from build123d import *

# Parameters (mm, degrees)
F2_R     = 3
F3_R     = 3
F4_R     = 7.243967
F5_DEPTH = 105.41


with BuildPart() as f1:
    # F0 (on Front) → F1 (revolve)
    with BuildSketch(Plane.XZ):
        Polygon((-12.904838, 16.591936), (-12.904838, 31.709034), (-12.904838, 46.826132), (-25.809675, 46.826132), (-25.809675, 56.412581), (-41.295484, 56.412581), (-41.295484, 63.418068), (-48.669677, 63.418068), (-48.669677, 49.038392), (-43.692097, 49.038392), (-43.692097, 31.709034), (-43.692097, 14.379676), (-48.669677, 14.379676), (-48.669677, 0), (-41.295484, 0), (-41.295484, 7.005487), (-25.809675, 7.005487), (-25.809675, 16.591936), align=None)
    revolve(axis=Axis((0, 0, 52.264599), (0, 0, 1)))

    # F2
    f2_edges = [f1.edges().sort_by_distance(p)[0] for p in [
        (43.692097, 0, 49.038392),
    ]]
    fillet(f2_edges, radius=F2_R)

    # F3
    f3_edges = [f1.edges().sort_by_distance(p)[0] for p in [
        (43.692097, 0, 14.379676),
    ]]
    fillet(f3_edges, radius=F3_R)

    # F4 (on Top) → F5 (cut)
    with BuildSketch(Plane.XY):
        with Locations((0, -33.43946)):
            Circle(F4_R)
        with Locations((-31.89178, -10.055439)):
            Circle(F4_R)
        with Locations((-19.180086, 27.392002)):
            Circle(F4_R)
        with Locations((20.356653, 26.529307)):
            Circle(F4_R)
        with Locations((31.422813, -11.436969)):
            Circle(F4_R)
    extrude(amount=F5_DEPTH, mode=Mode.SUBTRACT)


solid = f1.part
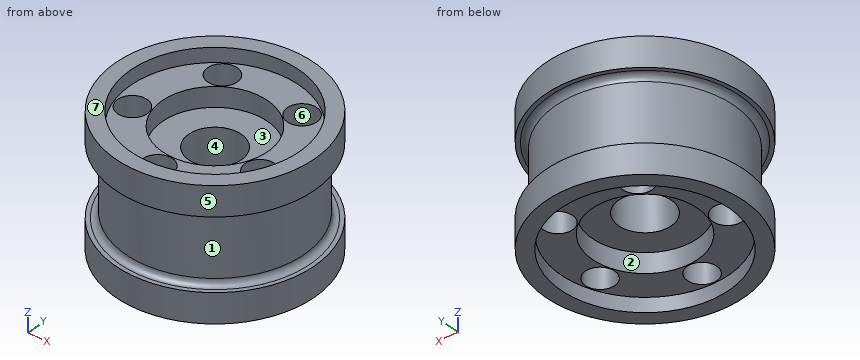
Could you check a few things on this model? Use its own coordinates, in mm. Face numbers are marked on the shaded views. A direction names the side the tool comes from. Give positions to 0.01 mm unless a question says otherwise; leave off trailing zeros. Order: outer loops, then holes, each group sorted by start corner. A loop starts at its lowest first (then second) coordinate and runs counter-clockwise, first axis right, second up.
1. I need wall thicknesses on L1, parallel to Y at x = 0, z = 52; L2, parallel to Y at x = 0, z = 59; L3, parallel to Y at x = 0, z = 23. Which ranges of each line are inside material? Lowest first, please.
2. Suppose I cut it at A-A (x = 0). Give the number of separate pieces and of enclosed holes in the cut face, plus the area to 3 significant figures.
3. We'd pull the mould along Y, two halves only. Please class the marked faces 5, 6 and 7: pulls with the +Y half, pulls with the -Y half, needs draft (parallel to the pull), parting line crosses it, or undercut.
4. For the marked faces 1, 2, 3 and 4, which set-ups out of +Z, -Z, +X, -X, +Y, -Y let a thin tool reach every point of the face, with its end or its side?
5. Will these pins go through, and if not, where does the flat tip stop? P1, Ø10, axis at y = 14.5, z = 28.5, coming from the -X side; P2, Ø13, axis at x = -31.89, y = -10.06, coming from the -Z side; P3, Ø1, axis at x = -16, z = 7.5, coming from the -Y side; P4, Ø10, axis at y = -31.5, z = 30.5, coming from the +X side.
6. Suppose I cut it at C-C (z = 32). List the corners of the cut face in (x, y) for me, plus the area to 3 significant figures.
7. Suppose I cut it at B-B (z = 4). List the corners of the cut face in (x, y) for me.
Solved:
1. L1: y = -48.67 to -40.68, -26.2 to -25.81, 25.81 to 48.67
1. L2: y = -48.67 to -41.3, 41.3 to 48.67
1. L3: y = -43.69 to -40.68, -26.2 to -12.9, 12.9 to 43.69
2. separate pieces: 3
2. enclosed holes: 0
2. area: 2,190 mm2
3. face 5: parting line crosses it
3. face 6: undercut
3. face 7: needs draft
4. face 1: none
4. face 2: -Z
4. face 3: +Z
4. face 4: +Z, -Z
5. P1: stops at x = -42.65
5. P2: passes through
5. P3: stops at y = -46.14
5. P4: stops at x = 34.74
6. outline: circle Ø87.38 at (0, 0); hole circle Ø14.49 at (-31.89, -10.06); hole circle Ø14.49 at (-19.18, 27.39); hole circle Ø25.81 at (0, 0); hole circle Ø14.49 at (0, -33.44); hole circle Ø14.49 at (20.36, 26.53); hole circle Ø14.49 at (31.42, -11.44)
6. area: 4,650 mm2
7. outline: circle Ø97.34 at (0, 0); hole circle Ø82.59 at (0, 0)
